Input: part model. Units: mm. Frame: model coordinates. Give positions to 0.01 mm unless a question says otherwise; leave off trailing zeros. Loops run counter-clockwise (first coordinate to the right, second up) from the corner with the lowest first, then second, coordinate; pieces in that order, holes last. Notation, with made-up numbers: (-22.5, 74) -> (22.5, 74) arc R16 ccw to (22.5, 95) -> close; hole circle Ø6 at (4.25, 42.5). An arc over 180 degrees is marked (long way). Use CSV: the item, a comma, the result in double quotes.
```python
from build123d import *

# Parameters (mm, degrees)
F0_R      = 1
F0_R_2    = 2
F0_R_3    = 4
F1_DEPTH  = 5
F2_DEPTH  = 7
F3_DEPTH  = 6.604
F4_R      = 1
F5_DEPTH  = 5
F6_R      = 1
F7_DEPTH  = 5
F8_R      = 1
F9_DEPTH  = 5
F10_R     = 1
F11_DEPTH = 5
F13_DEPTH = 3


with BuildPart() as f1:
    # F0 (on Front) → F1 (new body)
    with BuildSketch(Plane.XZ):
        Polygon((-75.6474129446, -7.9146586359), (-75.6474129446, -37.9146586359), (94.3547870554, -37.9146586359), (94.3547870554, 22.0853413641), (59.3547870554, 22.0853413641), (24.3525870554, 22.0853413641), (-75.6474129446, 22.0853413641), align=None)
        with Locations((-65.6474129446, -27.9146586359)):
            Circle(F0_R, mode=Mode.SUBTRACT)
        with Locations((-42.6474129446, -29.4146586359)):
            Circle(F0_R_2, mode=Mode.SUBTRACT)
        with Locations((24.3525870554, -29.4146586359)):
            Circle(F0_R_2, mode=Mode.SUBTRACT)
        with Locations((84.3547870554, -27.9146586359)):
            Circle(F0_R, mode=Mode.SUBTRACT)
        Polygon((59.3547870554, -0.9864554056), (65.3547870554, -4.4505570207), (65.3547870554, -11.378760251), (59.3547870554, -14.8428618661), (53.3547870554, -11.378760251), (53.3547870554, -4.4505570207), align=None, mode=Mode.SUBTRACT)
        with Locations((-65.6474129446, 12.0853413641)):
            Circle(F0_R, mode=Mode.SUBTRACT)
        with Locations((-42.6474129446, 13.5853413641)):
            Circle(F0_R_2, mode=Mode.SUBTRACT)
        with Locations((24.3525870554, 13.5853413641)):
            Circle(F0_R_2, mode=Mode.SUBTRACT)
        with Locations((84.3547870554, 12.0853413641)):
            Circle(F0_R, mode=Mode.SUBTRACT)
        Polygon((65.3547870554, -11.378760251), (65.3547870554, -4.4505570207), (59.3547870554, -0.9864554056), (53.3547870554, -4.4505570207), (53.3547870554, -11.378760251), (59.3547870554, -14.8428618661), align=None)
        with Locations((59.3547870554, -7.9146586359)):
            Circle(F0_R_3, mode=Mode.SUBTRACT)
        with Locations((24.3525870554, -29.4146586359)):
            Circle(F0_R_2)
        with Locations((24.3525870554, -29.4146586359)):
            Circle(F0_R, mode=Mode.SUBTRACT)
        with Locations((-42.6474129446, -29.4146586359)):
            Circle(F0_R_2)
        with Locations((-42.6474129446, -29.4146586359)):
            Circle(F0_R, mode=Mode.SUBTRACT)
        with Locations((-42.6474129446, 13.5853413641)):
            Circle(F0_R_2)
        with Locations((-42.6474129446, 13.5853413641)):
            Circle(F0_R, mode=Mode.SUBTRACT)
        with Locations((24.3525870554, 13.5853413641)):
            Circle(F0_R_2)
        with Locations((24.3525870554, 13.5853413641)):
            Circle(F0_R, mode=Mode.SUBTRACT)
        with Locations((24.3525870554, -29.4146586359)):
            Circle(F0_R)
        with Locations((-42.6474129446, -29.4146586359)):
            Circle(F0_R)
        with Locations((-42.6474129446, 13.5853413641)):
            Circle(F0_R)
        with Locations((24.3525870554, 13.5853413641)):
            Circle(F0_R)
    extrude(amount=F1_DEPTH)

    # F0 (on Front) → F2 (join)
    with BuildSketch(Plane.XZ):
        with Locations((-42.6474129446, 13.5853413641)):
            Circle(F0_R_2)
        with Locations((-42.6474129446, 13.5853413641)):
            Circle(F0_R, mode=Mode.SUBTRACT)
        with Locations((-42.6474129446, -29.4146586359)):
            Circle(F0_R_2)
        with Locations((-42.6474129446, -29.4146586359)):
            Circle(F0_R, mode=Mode.SUBTRACT)
        with Locations((24.3525870554, -29.4146586359)):
            Circle(F0_R_2)
        with Locations((24.3525870554, -29.4146586359)):
            Circle(F0_R, mode=Mode.SUBTRACT)
        with Locations((24.3525870554, 13.5853413641)):
            Circle(F0_R_2)
        with Locations((24.3525870554, 13.5853413641)):
            Circle(F0_R, mode=Mode.SUBTRACT)
        with Locations((-42.6474129446, -29.4146586359)):
            Circle(F0_R)
        with Locations((-42.6474129446, 13.5853413641)):
            Circle(F0_R)
        with Locations((24.3525870554, 13.5853413641)):
            Circle(F0_R)
        with Locations((24.3525870554, -29.4146586359)):
            Circle(F0_R)
    extrude(amount=F2_DEPTH)

    # F0 (on Front) → F3 (join)
    with BuildSketch(Plane.XZ):
        with Locations((-42.6474129446, 13.5853413641)):
            Circle(F0_R)
        with Locations((24.3525870554, 13.5853413641)):
            Circle(F0_R)
        with Locations((-42.6474129446, -29.4146586359)):
            Circle(F0_R)
    extrude(amount=F3_DEPTH)

    # F4 (on face) → F5 (cut)
    with BuildSketch(Plane.XZ.offset(7)):
        with Locations((-42.6474129446, 13.5853413641)):
            Circle(F4_R)
    extrude(amount=-F5_DEPTH, mode=Mode.SUBTRACT)

    # F6 (on face) → F7 (cut)
    with BuildSketch(Plane.XZ.offset(7)):
        with Locations((24.3525870554, 13.5853413641)):
            Circle(F6_R)
    extrude(amount=-F7_DEPTH, mode=Mode.SUBTRACT)

    # F8 (on face) → F9 (cut)
    with BuildSketch(Plane.XZ.offset(7)):
        with Locations((-42.6474129446, -29.4146586359)):
            Circle(F8_R)
    extrude(amount=-F9_DEPTH, mode=Mode.SUBTRACT)

    # F10 (on face) → F11 (cut)
    with BuildSketch(Plane.XZ.offset(7)):
        with Locations((24.3525870554, -29.4146586359)):
            Circle(F10_R)
    extrude(amount=-F11_DEPTH, mode=Mode.SUBTRACT)

    # F12 (on face) → F13 (cut)
    with BuildSketch(Plane.XZ.offset(5)):
        Polygon((65.3547870554, -11.378760251), (65.3547870554, -4.4505570207), (59.3547870554, -0.9864554056), (53.3547870554, -4.4505570207), (53.3547870554, -11.378760251), (59.3547870554, -14.8428618661), align=None)
    extrude(amount=-F13_DEPTH, mode=Mode.SUBTRACT)


solid = f1.part
```
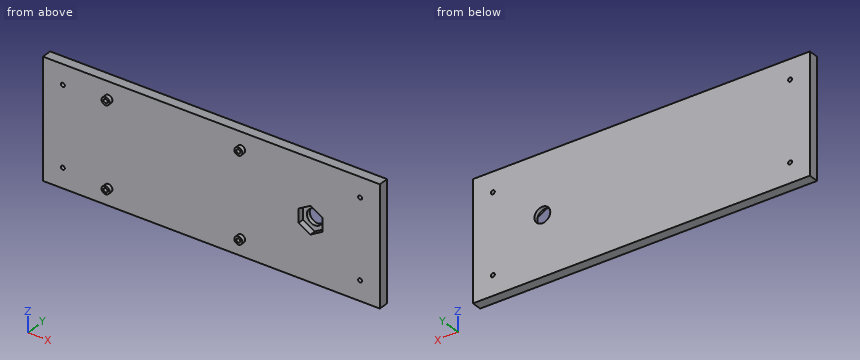
1) Section query B-B (z = 2). Return loops of the section in (x, y), then the cut area to 3 significant figures.
From the geometry:
outline,"(-75.65, -5) -> (94.35, -5) -> (94.35, 0) -> (-75.65, 0) -> close"
area,"850 mm^2"
2) Contact query for flat-ended pins moving along their axis: pin 1 (8 mm diameter, centred on x = -11.5, z = -2.5, fed in from -Y); pin 2 (1 mm diameter, centred on x = 24.5, z = -29.5, fed in from -Y). Output: stop coordinate, or through.
From the geometry:
pin 1,"stops at y = -5"
pin 2,"stops at y = -2"
3) Section query A-A (x = 12.5). Return loops of the section in (y, z).
From the geometry:
outline,"(-5, -37.91) -> (0, -37.91) -> (0, 22.09) -> (-5, 22.09) -> close"
4) Ray query, line 1 (Z direction, x = -65.5, y = -1.5); line 2 (Y direction, x = 38.5, z = 19.5); line 3 (X direction, y = -4.75, z = -12). Return the intervals inside material, ascending.
From the geometry:
line 1,"z = -37.91 to -28.9, -26.93 to 11.1, 13.07 to 22.09"
line 2,"y = -5 to 0"
line 3,"x = -75.65 to 54.43, 64.28 to 94.35"
